CAD build for the part. Positions are in the model's coordinates, mm. A direction names the side the tool comes from. Round coordinates to 2 decimals unless told otherwise and drop trailing zeros. Loops run counter-clockwise (first coordinate to the right, second up) from the corner with the lowest first, then second, coordinate; pieces in that order, holes last.
Autodesk Inventor part; units mm, degrees
ref_plane "YZ Plane" through (0, 0, 0) normal (1, 0, 0) x (0, 1, 0)
ref_plane "XZ Plane" through (0, 0, 0) normal (0, 1, 0) x (-1, 0, 0)
ref_plane "XY Plane" through (0, 0, 0) normal (0, 0, 1) x (1, 0, 0)
sketch "Sketch1" plane through (0, 0, 0) normal (0, 0, 1) x (1, 0, 0)
  line L0 (-34.0226, 19.6334) -> (65.9774, 19.6334)
  line L1 (65.9774, 19.6334) -> (65.9774, -20.3666)
  line L2 (65.9774, -20.3666) -> (-34.0226, -20.3666)
  line L3 (-34.0226, -20.3666) -> (-34.0226, 19.6334)
  point P0 (0, 0)
  dimension "d0" = 100
  dimension "d1" = 40
extrude "Extrusion1" add sketch "Sketch1" along normal blind 3.6
sketch "Sketch2" plane through (0, 0, 3.6) normal (0, 0, 1) x (1, 0, 0)
  line L0 (15.9774, -10.5166) -> (-24.0226, -10.5166)
  line L1 (-24.0226, -10.5166) -> (-24.0226, 9.7834)
  line L2 (-24.0226, 9.7834) -> (15.9774, 9.7834)
  line L3 (15.9774, 9.7834) -> (15.9774, -10.5166)
  line L4 (-34.0226, -20.3666) -> (65.9774, -20.3666)
  line L5 (65.9774, 19.6334) -> (-34.0226, 19.6334)
  line L6 (-34.0226, -20.3666) -> (-34.0226, 19.6334)
  point P0 (0, 0)
  dimension "d4" = 40
  dimension "d5" = 20.3
  dimension "d6" = 9.85
  dimension "d7" = 9.85
  dimension "d8" = 10
extrude "Extrusion2" cut sketch "Sketch2" against normal blind 4
sketch "Sketch3" plane through (0, 0, 3.6) normal (0, 0, 1) x (1, 0, 0)
  line L0 (65.9774, -20.3666) -> (65.9774, 19.6334)
  circle A0 centre (65.9774, -0.3666) radius 20
  point P0 (0, 0)
extrude "Extrusion3" add sketch "Sketch3" against normal blind 3.6
sketch "Sketch4" plane through (0, 0, 3.6) normal (0, 0, 1) x (1, 0, 0)
  arc A0 (65.9774, -20.3666) -> (65.9774, 19.6334) centre (65.9774, -0.3666) ccw
  circle A1 centre (65.9774, -0.3666) radius 5.25
  point P0 (0, 0)
  dimension "d13" = 10.5
extrude "Extrusion4" cut sketch "Sketch4" against normal blind 4
properties part number "plaat1"
Item 1: Flat gauge pins, fed straight in: P1, Ø1.1, axis at y = 4, z = 2, coming from the +X side; P2, Ø1.5, axis at x = 29.5, y = 14.5, coming from the -Z side; P3, Ø2, axis at y = -4, z = 3, coming from the +X side. Where does each tip first touch, or does it go through?
Answers follow:
P1: stops at x = 85.61
P2: stops at z = 0
P3: stops at x = 85.8
Item 2: Cut at C-C, the plane y = -4. Give the cut face in (x, z).
Answers follow:
outline: (-34.02, 0) - (-24.02, 0) - (-24.02, 3.6) - (-34.02, 3.6) - close; (15.98, 0) - (62.19, 0) - (62.19, 3.6) - (15.98, 3.6) - close; (69.77, 0) - (85.64, 0) - (85.64, 3.6) - (69.77, 3.6) - close
Item 3: 3-axis set-ups, long thin cutter, end or side, ignore diameter. For faces 4 (the flat face through (-4, -10.517, 2)), 5 (the flat face through (25, 0, 0)): which of +Z, -Z, +X, -X, +Y, -Y reach the whole face in a straight line?
Answers follow:
face 4: +Z, -Z
face 5: -Z, +X, -X, +Y, -Y
Item 4: Probe line 1 (X direction, y = 0, z = 1.65); line 2 (Y direction, x = -12.5, z = 1.2); line 3 (X direction, y = 2, z = 1.8). List the from-to ranges inside material, lowest first.
Answers follow:
line 1: x = -34.02 to -24.02, 15.98 to 60.74, 71.21 to 85.97
line 2: y = -20.37 to -10.52, 9.78 to 19.63
line 3: x = -34.02 to -24.02, 15.98 to 61.29, 70.66 to 85.84
Item 5: Cut at D-D, the plane z = 2.8. Give the cut face in (x, y).
Answers follow:
outline: (-34.02, -20.37) - (65.98, -20.37) arc R20 ccw to (65.98, 19.63) - (-34.02, 19.63) - close; hole (-24.02, -10.52) - (15.98, -10.52) - (15.98, 9.78) - (-24.02, 9.78) - close; hole circle Ø10.5 at (65.98, -0.37)
Item 6: Cut at A-A, the plane x = -12.5. Give the cut face in (y, z).
Answers follow:
outline: (-20.37, 0) - (-10.52, 0) - (-10.52, 3.6) - (-20.37, 3.6) - close; (9.78, 0) - (19.63, 0) - (19.63, 3.6) - (9.78, 3.6) - close
Item 7: Cut at B-B, the plane y = 7. Give the cut face in (x, z).
Answers follow:
outline: (-34.02, 0) - (-24.02, 0) - (-24.02, 3.6) - (-34.02, 3.6) - close; (15.98, 0) - (84.57, 0) - (84.57, 3.6) - (15.98, 3.6) - close
Item 8: Two-plate mould, pull along Y, no slides. Class faces 1 (the flat face through (-34.023, -1, 2)), 2 (the cylindrical face through (60.732, -0.136, 1.825)), 3 (the flat face through (17, -20.367, 2)): released by +Y, released by -Y, zero draft, split by the parting line, or undercut.
Answers follow:
face 1: zero draft
face 2: undercut
face 3: released by -Y
